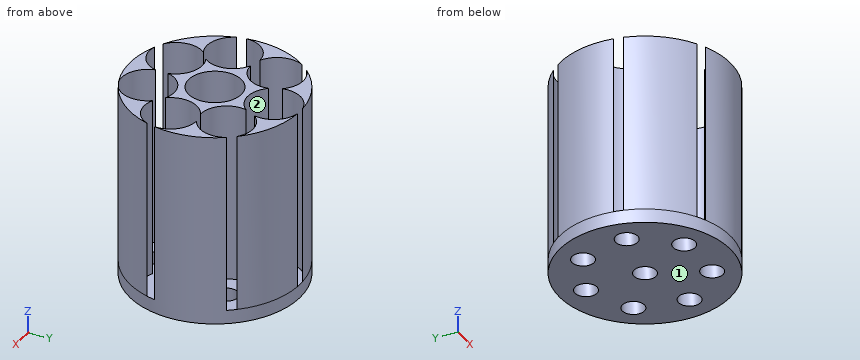
from build123d import *

# Parameters (mm, degrees)
F1_DEPTH = 65
F0_R     = 9.6
F2_R     = 31
F2_R_2   = 9.6
F3_DEPTH = 5
F5_D     = 8


with BuildPart() as f1:
    # F0 (on Top) → F1 (new body)
    with BuildSketch(Plane.XY):
        with BuildLine():
            ThreePointArc((0, -21.6377846635), (-4.4866514155, -27.6603721731), (-11.936497657, -28.6097889486))
            ThreePointArc((-11.936497657, -28.6097889486), (0, -31), (11.936497657, -28.6097889486))
            ThreePointArc((11.936497657, -28.6097889486), (4.4866514155, -27.6603721731), (0, -21.6377846635))
        make_face()
    extrude(amount=F1_DEPTH)



with BuildPart() as f1b:
    # F0 (on Top) → F1, piece 2 (new body)
    with BuildSketch(Plane.XY):
        with BuildLine():
            ThreePointArc((7.421093957, 15.4100603877), (0, 11.9), (-7.421093957, 15.4100603877))
            ThreePointArc((-7.421093957, 15.4100603877), (-9.3037946414, 7.4195286421), (-16.6750467587, 3.8059706078))
            ThreePointArc((-16.6750467587, 3.8059706078), (-11.601642155, -2.6479991141), (-13.3723492421, -10.6640926674))
            ThreePointArc((-13.3723492421, -10.6640926674), (-5.1632164955, -10.721529528), (0, -17.1038766563))
            ThreePointArc((0, -17.1038766563), (5.1632164955, -10.721529528), (13.3723492421, -10.6640926674))
            ThreePointArc((13.3723492421, -10.6640926674), (11.601642155, -2.6479991141), (16.6750467587, 3.8059706078))
            ThreePointArc((16.6750467587, 3.8059706078), (9.3037946414, 7.4195286421), (7.421093957, 15.4100603877))
        make_face()
        Circle(F0_R, mode=Mode.SUBTRACT)
    extrude(amount=F1_DEPTH)


with BuildPart() as f1c:
    # F0 (on Top) → F1, piece 3 (new body)
    with BuildSketch(Plane.XY):
        with BuildLine():
            ThreePointArc((-23.1677349851, 20.5974769246), (-16.0437189504, 22.9744491102), (-9.388282916, 19.4949703522))
            ThreePointArc((-9.388282916, 19.4949703522), (-7.9590524573, 26.8678192948), (-1.6589094237, 30.9555813953))
            ThreePointArc((-1.6589094237, 30.9555813953), (-13.4503959126, 27.930034905), (-23.1677349851, 20.5974769246))
        make_face()
    extrude(amount=F1_DEPTH)


with BuildPart() as f1d:
    # F0 (on Top) → F1, piece 4 (new body)
    with BuildSketch(Plane.XY):
        with BuildLine():
            ThreePointArc((-30.5486024144, -5.2709477823), (-27.9652427562, 1.7808501523), (-21.0952802263, 4.8148600521))
            ThreePointArc((-21.0952802263, 4.8148600521), (-25.9684950295, 10.5291735468), (-25.2363612008, 18.0035016966))
            ThreePointArc((-25.2363612008, 18.0035016966), (-30.2227652776, 6.8981489526), (-30.5486024144, -5.2709477823))
        make_face()
    extrude(amount=F1_DEPTH)


with BuildPart() as f1e:
    # F0 (on Top) → F1, piece 5 (new body)
    with BuildSketch(Plane.XY):
        with BuildLine():
            ThreePointArc((-14.9257491478, -27.1702413014), (-18.8283683796, -20.7537652931), (-16.9171012608, -13.4909380725))
            ThreePointArc((-16.9171012608, -13.4909380725), (-24.4231311838, -13.738154638), (-29.8103182658, -8.5055819842))
            ThreePointArc((-29.8103182658, -8.5055819842), (-24.2367759565, -19.3281838576), (-14.9257491478, -27.1702413014))
        make_face()
    extrude(amount=F1_DEPTH)


with BuildPart() as f1f:
    # F0 (on Top) → F1, piece 6 (new body)
    with BuildSketch(Plane.XY):
        with BuildLine():
            ThreePointArc((29.8103182658, -8.5055819842), (24.4231311838, -13.738154638), (16.9171012608, -13.4909380725))
            ThreePointArc((16.9171012608, -13.4909380725), (18.8283683796, -20.7537652931), (14.9257491478, -27.1702413014))
            ThreePointArc((14.9257491478, -27.1702413014), (24.2367759565, -19.3281838576), (29.8103182658, -8.5055819842))
        make_face()
    extrude(amount=F1_DEPTH)


with BuildPart() as f1g:
    # F0 (on Top) → F1, piece 7 (new body)
    with BuildSketch(Plane.XY):
        with BuildLine():
            ThreePointArc((25.2363612008, 18.0035016966), (25.9684950295, 10.5291735468), (21.0952802263, 4.8148600521))
            ThreePointArc((21.0952802263, 4.8148600521), (27.9652427562, 1.7808501523), (30.5486024144, -5.2709477823))
            ThreePointArc((30.5486024144, -5.2709477823), (30.2227652776, 6.8981489526), (25.2363612008, 18.0035016966))
        make_face()
    extrude(amount=F1_DEPTH)


with BuildPart() as f1h:
    # F0 (on Top) → F1, piece 8 (new body)
    with BuildSketch(Plane.XY):
        with BuildLine():
            ThreePointArc((1.6589094237, 30.9555813953), (7.9590524573, 26.8678192948), (9.388282916, 19.4949703522))
            ThreePointArc((9.388282916, 19.4949703522), (16.0437189504, 22.9744491102), (23.1677349851, 20.5974769246))
            ThreePointArc((23.1677349851, 20.5974769246), (13.4503959126, 27.930034905), (1.6589094237, 30.9555813953))
        make_face()
    extrude(amount=F1_DEPTH)


with BuildPart() as f1_1:
    add(f1.part)

    add(f1b.part)  # F3 merges F1b

    add(f1c.part)  # F3 merges F1c

    add(f1d.part)  # F3 merges F1d

    add(f1e.part)  # F3 merges F1e

    add(f1f.part)  # F3 merges F1f

    add(f1g.part)  # F3 merges F1g

    add(f1h.part)  # F3 merges F1h
    # F2 (on face) → F3 (join)
    with BuildSketch(Plane(origin=(0, 0, 0), x_dir=(1, 0, 0), z_dir=(0, 0, -1))):
        Circle(F2_R)
        with BuildLine():
            ThreePointArc((-13.3723492421, 10.6640926674), (-5.1632164955, 10.721529528), (0, 17.1038766563))
            ThreePointArc((0, 17.1038766563), (5.1632164955, 10.721529528), (13.3723492421, 10.6640926674))
            ThreePointArc((13.3723492421, 10.6640926674), (11.601642155, 2.6479991141), (16.6750467587, -3.8059706078))
            ThreePointArc((16.6750467587, -3.8059706078), (9.3037946414, -7.4195286421), (7.421093957, -15.4100603877))
            ThreePointArc((7.421093957, -15.4100603877), (0, -11.9), (-7.421093957, -15.4100603877))
            ThreePointArc((-7.421093957, -15.4100603877), (-9.3037946414, -7.4195286421), (-16.6750467587, -3.8059706078))
            ThreePointArc((-16.6750467587, -3.8059706078), (-11.601642155, 2.6479991141), (-13.3723492421, 10.6640926674))
        make_face(mode=Mode.SUBTRACT)
        with BuildLine():
            ThreePointArc((13.3723492421, 10.6640926674), (5.1632164955, 10.721529528), (0, 17.1038766563))
            ThreePointArc((0, 17.1038766563), (-5.1632164955, 10.721529528), (-13.3723492421, 10.6640926674))
            ThreePointArc((-13.3723492421, 10.6640926674), (-11.601642155, 2.6479991141), (-16.6750467587, -3.8059706078))
            ThreePointArc((-16.6750467587, -3.8059706078), (-9.3037946414, -7.4195286421), (-7.421093957, -15.4100603877))
            ThreePointArc((-7.421093957, -15.4100603877), (0, -11.9), (7.421093957, -15.4100603877))
            ThreePointArc((7.421093957, -15.4100603877), (9.3037946414, -7.4195286421), (16.6750467587, -3.8059706078))
            ThreePointArc((16.6750467587, -3.8059706078), (11.601642155, 2.6479991141), (13.3723492421, 10.6640926674))
        make_face()
        Circle(F2_R_2, mode=Mode.SUBTRACT)
        Circle(F2_R_2)
    extrude(amount=F3_DEPTH)

    # F5 (through all)
    with Locations(Plane.XY):
        with Locations((9.328500391, -19.3708306599), (20.9609501119, -4.7842000801), (16.8093768731, 13.40503074), (0, 21.5), (0, 0), (-16.8093768731, 13.40503074), (-20.9609501119, -4.7842000801), (-9.328500391, -19.3708306599)):
            Hole(F5_D / 2)


solid = f1_1.part
Can you work these out from the model? Positions are in its coordinate system, mm. Face numbers are marked on the shaded views. Coordinates: 2 decimals unless noted, no trailing zeros. Loops run counter-clockwise (first coordinate to the right, second up) from the corner with the lowest first, then second, coordinate; pieces in that order, holes last. Notation, with made-up numbers: (77, -28) - (113, -28) arc R38 cw to (113, 11) - close; hole circle Ø3 at (81, -24). An arc over 180 degrees is marked (long way). Answer as a JSON object with one key per item and string values. Group by question number.
Item 1: For pin 1 (10 mm diameter, centred on x = 7.5, z = 40.5, fed in from +Y); pin 2 (4 mm diameter, centred on y = 8.5, z = 44.5, fed in from -X); pin 3 (13 mm diameter, centred on x = -16.81, y = 13.41, fed in from -Z); pin 4 (6 mm diameter, centred on x = -0.5, z = 3.5, fed in from -Y), each with a flat end and sliding along its axis, tell me the tip position at first contact or that it passes through.
Item 2: If we section it at C-C (y = 21.5): List the corners of the cut face in (x, z) for me.
Item 3: If we section it at B-B (y = -7): List the corners of the cut face in (x, z) for me, plus the area to 3 significant figures.
Item 4: If I drill on L1, parallel to Y at x = -22, z = 54.5; L2, parallel to Y at x = -5.5, z = 38; L3, parallel to X at y = -2.5, z = 25, over which ranges is the centre line in solid material (lowest first)? Write a range as from..to.
Item 5: If we section it at A-A (z = 39.5): State how many separate pieces and enclosed holes the cut face has, plus the area to 3 significant figures.
Item 6: If we mould it in two halves opening along Y, with no side actions, what happens to the marked faces 1 and 2? For each: released by +Y, released by -Y, zero draft, split by the parting line, or undercut.
Returned:
{
 "1": {"pin 1": "stops at y = 30.9", "pin 2": "stops at x = -30.31", "pin 3": "stops at z = -5", "pin 4": "stops at y = -31"},
 "2": {"outline": "(-22.33, -5) - (-4, -5) - (-4, 0) - (-9.6, 0) - (-9.6, 65) - (-11.65, 65) - (-11.65, 0) - (-21.97, 0) - (-21.97, 65) - (-22.33, 65) - close; (4, -5) - (22.33, -5) - (22.33, 65) - (21.97, 65) - (21.97, 0) - (11.65, 0) - (11.65, 65) - (9.6, 65) - (9.6, 0) - (4, 0) - close"},
 "3": {"outline": "(-30.2, -5) - (-24.29, -5) - (-24.29, 0) - (-30.2, 0) - close; (-17.63, -5) - (17.63, -5) - (17.63, 0) - (11.62, 0) - (11.62, 65) - (6.57, 65) - (6.57, 0) - (-6.57, 0) - (-6.57, 65) - (-11.62, 65) - (-11.62, 0) - (-17.63, 0) - close; (24.29, -5) - (30.2, -5) - (30.2, 0) - (24.29, 0) - close", "area": "892 mm²"},
 "4": {"L1": "y = -21.84..-14.33, 4.76..5.33, 21.48..21.84", "L2": "y = -30.51..-28.17, -10.57..-7.87, 7.87..13.63, 29.37..30.51", "L3": "x = -30.9..-30.29, -11.64..-9.27, 9.27..11.64, 30.29..30.9"},
 "5": {"separate pieces": "8", "enclosed holes": "1", "area": "716 mm²"},
 "6": {"face 1": "zero draft", "face 2": "undercut"}
}
